Part model, mm, in its own coordinate system. A direction names the side the tool comes from. Coordinates: 2 decimals unless noted, no trailing zeros. Loops run counter-clockwise (first coordinate to the right, second up) from the corner with the lowest first, then second, coordinate; pieces in that order, holes last. Notation, with made-up numbers: (15, 14.25) - (65, 14.25) arc R26 cw to (65, 31.25) - close; hole circle Ø8 at (6.25, 24.25). An arc over 180 degrees is marked (long way). Answer as CSV lines item,"result".
from build123d import *

# Parameters (mm, degrees)
SKETCH1_R               = 11.43
BOSS_EXTRUDE1_DEPTH     = 4.7625
MIRROR2_COPY_1_SKETCH_R = 11.43
MIRROR2_COPY_1_DEPTH    = 4.7625
M4_CLEARANCE_HOLE2_D    = 4.5


with BuildPart() as part:
    # Sketch1 → Boss-Extrude1 (new body)
    with BuildSketch(Plane.XY):
        with BuildLine():
            Line((33.9979, -29.3751), (33.9979, 36.9951))
            Line((33.9979, 36.9951), (-33.9979, 36.9951))
            Line((-33.9979, 36.9951), (-33.9979, -36.9951))
            Line((-33.9979, -36.9951), (26.3779, -36.9951))
            Line((26.3779, -36.9951), (29.48387433, -40.10107433))
            ThreePointArc((29.48387433, -40.10107433), (37.10387433, -40.10107433), (37.10387433, -32.48107433))
            Line((37.10387433, -32.48107433), (33.9979, -29.3751))
        make_face()
        Circle(SKETCH1_R, mode=Mode.SUBTRACT)
        Polygon((33.926365892, -36.9951), (33.9979, -36.923565892), (33.9979, -36.9951), align=None, mode=Mode.SUBTRACT)
    boss_extrude1 = extrude(amount=BOSS_EXTRUDE1_DEPTH)

    # Mirror1: Boss-Extrude1 across plane
    add(boss_extrude1.mirror(Plane.ZX))

    # Mirror2: Boss-Extrude1 across plane
    add(boss_extrude1.mirror(Plane(origin=(0, 0, 0), x_dir=(0, 0, 1), z_dir=(1, 0, 0))))

    # Mirror2 copy 1 sketch → Mirror2 copy 1 (add)
    with BuildSketch(Plane(origin=(0, 0, 0), x_dir=(-1, 0, 0), z_dir=(0, 0, 1))):
        with BuildLine():
            Line((33.9979, -29.3751), (33.9979, 36.9951))
            Line((33.9979, 36.9951), (-33.9979, 36.9951))
            Line((-33.9979, 36.9951), (-33.9979, -36.9951))
            Line((-33.9979, -36.9951), (26.3779, -36.9951))
            Line((26.3779, -36.9951), (29.48387433, -40.10107433))
            ThreePointArc((29.48387433, -40.10107433), (37.10387433, -40.10107433), (37.10387433, -32.48107433))
            Line((37.10387433, -32.48107433), (33.9979, -29.3751))
        make_face()
        Circle(MIRROR2_COPY_1_SKETCH_R, mode=Mode.SUBTRACT)
        Polygon((33.926365892, -36.9951), (33.9979, -36.923565892), (33.9979, -36.9951), align=None, mode=Mode.SUBTRACT)
    extrude(amount=MIRROR2_COPY_1_DEPTH)

    # M4 Clearance Hole2 (through all)
    with Locations(Plane.XY.offset(4.7625)):
        with Locations((-33.29387433, 36.29107433), (33.29387433, 36.29107433), (32.547164682, -36.586652732), (-33.29387433, -36.29107433)):
            Hole(M4_CLEARANCE_HOLE2_D / 2)


solid = part.part
Q1. Flat gauge pins, fed straight in: pin 1 (1.4 mm diameter, centred on x = 1.5, z = 3, fed in from +Y); pin 2 (1 mm diameter, centred on x = 27, z = 3, fed in from +Y); pin 3 (12 mm diameter, centred on x = 24.5, y = -1, fed in from -Z); pin 4 (2.5 mm diameter, centred on y = -11.5, z = 1.5, fed in from -X). Where does each tip first touch, or does it go through?
Results:
pin 1,"stops at y = 37"
pin 2,"stops at y = 38.12"
pin 3,"stops at z = 0"
pin 4,"stops at x = -34"
Q2. Saw through at A-A (x = 0). Give the cut face in (y, z), then the cut area to 3 significant figures.
Results:
outline,"(-37, 0) - (-11.43, 0) - (-11.43, 4.76) - (-37, 4.76) - close; (11.43, 0) - (37, 0) - (37, 4.76) - (11.43, 4.76) - close"
area,"244 mm^2"
Q3. Which spindle directions (+Z, -Z, +X, -X, +Y, -Y) get a long thin tool onto all of the face, cutting with end or side? Do faces 1 (the face through (-35.57, -30.95, 2.35)), 2 (the face through (27.91, 38.53, 2.35)), 3 (the face through (37, -40.2, 2.3)), 4 (the face through (35.57, -30.95, 2.35)), 5 (the face through (0, -36.995, 2)). Say none if no direction does.
Results:
face 1,"+Z, -Z, -X"
face 2,"+Z, -Z, +Y"
face 3,"+Z, -Z"
face 4,"+Z, -Z, +X"
face 5,"+Z, -Z, -Y"
Q4. Wall check: L1, parallel to X at y = -36.5, z = 2.8; L2, parallel to X at y = 36, z = 2.2; L3, parallel to X at y = 0, z = 2.4. Give the ranges that are in metal, low to high.
Results:
L1,"x = -38.68 to -35.53, -31.05 to 30.3, 34.8 to 38.68"
L2,"x = -38.67 to -35.52, -31.06 to 31.06, 35.52 to 38.67"
L3,"x = -34 to -11.43, 11.43 to 34"
Q5. Saw through at D-D (y = 12.5). Give the cut face in (x, z).
Results:
outline,"(-34, 0) - (34, 0) - (34, 4.76) - (-34, 4.76) - close"
Q6. Two-plate mould, pull along X, no slides. Class faces 6 (the face through (8, -9, 0)), 7 (the face through (-34.33, -38.29, 2.35)), 8 (the face through (-35.57, 30.95, 2.35)): released by +X, released by -X, zero draft, split by the parting line, or undercut.
Results:
face 6,"zero draft"
face 7,"undercut"
face 8,"released by -X"
Q7. Saw through at B-B (y = 0). Give the cut face in (x, z), then the cut area to 3 significant figures.
Results:
outline,"(-34, 0) - (-11.43, 0) - (-11.43, 4.76) - (-34, 4.76) - close; (11.43, 0) - (34, 0) - (34, 4.76) - (11.43, 4.76) - close"
area,"215 mm^2"
Q8. Saw through at C-C (z = 3.85). Give the cut face in (x, y), then the cut area to 3 significant figures.
Results:
outline,"(-37.1, -32.48) arc R5.39 ccw to (-29.48, -40.1) - (-26.38, -37) - (26.38, -37) - (29.48, -40.1) arc R5.39 ccw to (37.1, -32.48) - (34, -29.38) - (34, 29.38) - (37.1, 32.48) arc R5.39 ccw to (29.48, 40.1) - (26.38, 37) - (-26.38, 37) - (-29.48, 40.1) arc R5.39 ccw to (-37.1, 32.48) - (-34, 29.38) - (-34, -29.38) - close; hole circle Ø4.5 at (-33.29, -36.29); hole circle Ø4.5 at (-33.29, 36.29); hole circle Ø22.86 at (0, 0); hole circle Ø4.5 at (32.55, -36.59); hole circle Ø4.5 at (33.29, 36.29)"
area,"4,810 mm^2"
